Could you check a few things on this model? Use its own coordinates, in mm. Face numbers are marked on the shaded views. A direction names the side the tool comes from. Coordinates: 2 decimals unless noted, no trailing zeros. Write each loop counter-clockwise with the first axis right and the second up, starting at its lowest first coordinate (ties: lowest second). Pieces come first, ordered by that corner, then holes. Notation, with made-up numbers: (17.5, 78.5) - (43.5, 78.5) arc R15 cw to (43.5, 98.5) - close; hole circle Ø5 at (14, 56). An arc over 180 degrees is marked (long way). Write item = value, one per line. Start each with the question number.
```python
from build123d import *

# Parameters (mm, degrees)
BOX007_W          = 4.3
BOX007_H          = 5
BOX007_DEPTH      = 2
CHAMFER001_SIZE   = 1.5
BOX006_W          = 4.3
BOX006_H          = 5
BOX006_DEPTH      = 2
CHAMFER_SIZE      = 1.5
BOX003_W          = 10
BOX003_H          = 10
BOX003_DEPTH      = 40
BOX002_W          = 10
BOX002_H          = 10
BOX002_DEPTH      = 40
CYLINDER010_R     = 3.5
CYLINDER010_DEPTH = 35.7
CYLINDER008_R     = 4.6
CYLINDER008_DEPTH = 22
CYLINDER006_R     = 1.85
CYLINDER006_DEPTH = 10
CYLINDER003_R     = 1.7
CYLINDER003_DEPTH = 50
CYLINDER002_R     = 1.7
CYLINDER002_DEPTH = 50
CYLINDER_R        = 1.5
CYLINDER_DEPTH    = 10
BOX001_W          = 10
BOX001_H          = 6
BOX001_DEPTH      = 3
FILLET_R          = 2.5
FILLET001_R       = 2.5
BOX_W             = 65
BOX_H             = 22
BOX_DEPTH         = 18.5


with BuildPart() as chamfer001:
    # Box007 → Box007 (new body)
    with BuildSketch(Plane(origin=(41, -2.5, 17.53), x_dir=(1, 0, 0), z_dir=(0, 0, 1))):
        with Locations((2.15, 2.5)):
            Rectangle(BOX007_W, BOX007_H)
    extrude(amount=BOX007_DEPTH)

    # Chamfer001
    chamfer001_edges = [chamfer001.edges().sort_by_distance(p)[0] for p in [
        (45.3, 0, 19.53),
    ]]
    chamfer(chamfer001_edges, length=CHAMFER001_SIZE)


with BuildPart() as part_mirroring:
    # Part__Mirroring: instance of Chamfer001
    add(chamfer001.part.mirror(Plane(origin=(0, 0, 0), x_dir=(0, 1, 0), z_dir=(0, 0, 1))))


with BuildPart() as part_mirroring_1:
    # Part__Mirroring placement: moved
    add(part_mirroring.part.moved(Location((0, 0, 18.4))))


with BuildPart() as fusion004:
    # Box006 → Box006 (new body)
    with BuildSketch(Plane(origin=(41, -2.5, 17.53), x_dir=(1, 0, 0), z_dir=(0, 0, 1))):
        with Locations((2.15, 2.5)):
            Rectangle(BOX006_W, BOX006_H)
    extrude(amount=BOX006_DEPTH)

    # Chamfer
    chamfer_edges = [fusion004.edges().sort_by_distance(p)[0] for p in [
        (45.3, 0, 19.53),
    ]]
    chamfer(chamfer_edges, length=CHAMFER_SIZE)

    # Fusion004: union Part__Mirroring
    add(part_mirroring_1.part)


with BuildPart() as cube003:
    # Box003 → Box003 (new body)
    with BuildSketch(Plane(origin=(-0.55, -5, 5), x_dir=(1, 0, 0), z_dir=(0, 0, 1))):
        with Locations((5, 5)):
            Rectangle(BOX003_W, BOX003_H)
    extrude(amount=BOX003_DEPTH)


with BuildPart() as cube002:
    # Box002 → Box002 (new body)
    with BuildSketch(Plane(origin=(11.75, -5, -11), x_dir=(1, 0, 0), z_dir=(0, 0, 1))):
        with Locations((5, 5)):
            Rectangle(BOX002_W, BOX002_H)
    extrude(amount=BOX002_DEPTH)


with BuildPart() as cut004:
    # Cylinder010 → Cylinder010 (new body)
    with BuildSketch(Plane(origin=(10.6, 0, -9), x_dir=(1, 0, 0), z_dir=(0, 0, 1))):
        Circle(CYLINDER010_R)
    extrude(amount=CYLINDER010_DEPTH)

    # Cut003: cut Cube002
    add(cube002.part, mode=Mode.SUBTRACT)

    # Cut004: cut Cube003
    add(cube003.part, mode=Mode.SUBTRACT)


with BuildPart() as cylinder004:
    # Cylinder008 → Cylinder008 (new body)
    with BuildSketch(Plane(origin=(10.6, 0, -2.8), x_dir=(1, 0, 0), z_dir=(0, 0, 1))):
        Circle(CYLINDER008_R)
    extrude(amount=CYLINDER008_DEPTH)


with BuildPart() as cylinder003:
    # Cylinder006 → Cylinder006 (new body)
    with BuildSketch(Plane(origin=(22, 0, 10.2), x_dir=(1, 0, 0), z_dir=(0, 0, 1))):
        Circle(CYLINDER006_R)
    extrude(amount=CYLINDER006_DEPTH)


with BuildPart() as cylinder002:
    # Cylinder003 → Cylinder003 (new body)
    with BuildSketch(Plane(origin=(31, -8.8, -25), x_dir=(1, 0, 0), z_dir=(0, 0, 1))):
        Circle(CYLINDER003_R)
    extrude(amount=CYLINDER003_DEPTH)


with BuildPart() as cylinder001:
    # Cylinder002 → Cylinder002 (new body)
    with BuildSketch(Plane(origin=(31, 8.8, -25), x_dir=(1, 0, 0), z_dir=(0, 0, 1))):
        Circle(CYLINDER002_R)
    extrude(amount=CYLINDER002_DEPTH)


with BuildPart() as cylinder:
    # Cylinder → Cylinder (new body)
    with BuildSketch(Plane(origin=(-2.8, 0, 3), x_dir=(1, 0, 0), z_dir=(0, 0, 1))):
        Circle(CYLINDER_R)
    extrude(amount=CYLINDER_DEPTH)


with BuildPart() as fillet001:
    # Box001 → Box001 (new body)
    with BuildSketch(Plane(origin=(-5, -3, 7), x_dir=(1, 0, 0), z_dir=(0, 0, 1))):
        with Locations((5, 3)):
            Rectangle(BOX001_W, BOX001_H)
    extrude(amount=BOX001_DEPTH)

    # Cut: cut Cylinder
    add(cylinder.part, mode=Mode.SUBTRACT)

    # Fillet
    fillet_edges = [fillet001.edges().sort_by_distance(p)[0] for p in [
        (-5, -3, 8.5),
    ]]
    fillet(fillet_edges, radius=FILLET_R)

    # Fillet001
    fillet001_edges = [fillet001.edges().sort_by_distance(p)[0] for p in [
        (-5, 3, 8.5),
    ]]
    fillet(fillet001_edges, radius=FILLET001_R)


with BuildPart() as motor:
    # Box → Box (new body)
    with BuildSketch(Plane(origin=(0, -11, 0), x_dir=(1, 0, 0), z_dir=(0, 0, 1))):
        with Locations((32.5, 11)):
            Rectangle(BOX_W, BOX_H)
    extrude(amount=BOX_DEPTH)

    # Fusion: union Fillet001
    add(fillet001.part)

    # Cut001: cut Cylinder001
    add(cylinder001.part, mode=Mode.SUBTRACT)

    # Cut002: cut Cylinder002
    add(cylinder002.part, mode=Mode.SUBTRACT)

    # Fusion001: union Cylinder003
    add(cylinder003.part)

    # Fusion002: union Cylinder004
    add(cylinder004.part)

    # Fusion003: union Cut004
    add(cut004.part)

    # Fusion006: union Fusion004
    add(fusion004.part)


with BuildPart() as motor_1:
    # Fusion006 placement: moved
    add(motor.part.moved(Location((-10.6, 0, 3))))


solid = motor_1.part
```
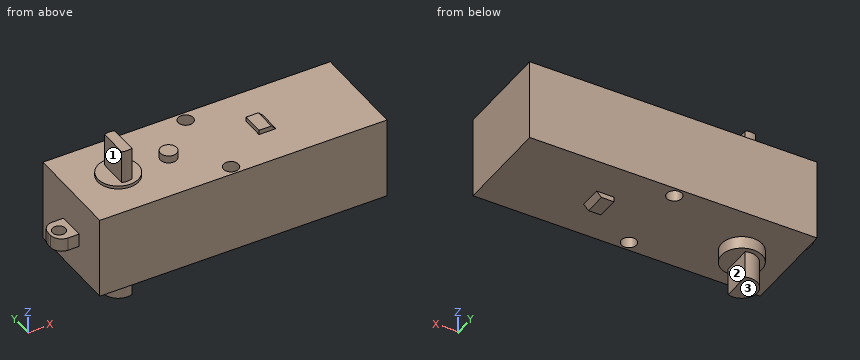
1) Suppose I cut it at A-A on y = -8.8. Please give me the cut outline in (x, z), plus the area to 3 significant figures.
2) If I drill on probe 1 along Y at (x, z) = (20.4, 10.5); probe 2 along X at (y, z) = (-8.8, 9); probe 3 along Z at (x, y) = (24, -8.5), over which ranges is the centre line in solid material (lowest first)? Write a range as [from, to].
3) Suppose I cut it at C-C on z = 7. Please give me the cut outline in (x, y), plus the area to 3 significant figures.
4) Which directions (+Z, -Z, +X, -X, +Y, -Y) give clear straight access to the entire face, cutting with the end or side of a thin tool? Please do the marked faces 1, 2 and 3.
5) For P1, Ø0.9, axis at x = 31.5, z = 2.5, coming from the -Y side; P2, Ø0.6, axis at x = 32.5, z = 2.5, coming from the +Y side; P3, Ø1.5, axis at x = 9, y = -1.5, coming from the +Z side, each with a flat end and sliding along its axis, tell me the tip position at first contact or that it passes through.
6) Suppose I cut it at D-D on x = 0. Please give me the cut outline in (y, z).
7) Suppose I cut it at B-B on x = 20.4. Please give me the cut outline in (y, z).
Reply:
q1.outline = (-10.6, 3) - (18.7, 3) - (18.7, 21.5) - (-10.6, 21.5) - close; (22.1, 3) - (54.4, 3) - (54.4, 21.5) - (22.1, 21.5) - close
q1.area = 1,140 mm^2
q2.probe_1 = [-11, -10.5], [-7.1, 7.1], [10.5, 11]
q2.probe_2 = [-10.6, 18.7], [22.1, 54.4]
q2.probe_3 = [3, 21.5]
q3.outline = (-10.6, -11) - (54.4, -11) - (54.4, 11) - (-10.6, 11) - close; hole circle Ø3.4 at (20.4, -8.8); hole circle Ø3.4 at (20.4, 8.8)
q3.area = 1,410 mm^2
q4.face_1 = +Z, -X, +Y, -Y
q4.face_2 = -Z, +X, +Y, -Y
q4.face_3 = -Z, +X, -X, +Y, -Y
q5.P1 = -2.5
q5.P2 = 2.5
q5.P3 = 21.5
q6.outline = (-11, 3) - (-4.6, 3) - (-4.6, 0.2) - (-3.5, 0.2) - (-3.5, -6) - (3.5, -6) - (3.5, 0.2) - (4.6, 0.2) - (4.6, 3) - (11, 3) - (11, 21.5) - (4.6, 21.5) - (4.6, 22.2) - (3.5, 22.2) - (3.5, 29.7) - (-3.5, 29.7) - (-3.5, 22.2) - (-4.6, 22.2) - (-4.6, 21.5) - (-11, 21.5) - close
q7.outline = (-11, 3) - (-10.5, 3) - (-10.5, 21.5) - (-11, 21.5) - close; (-7.1, 3) - (7.1, 3) - (7.1, 21.5) - (-7.1, 21.5) - close; (10.5, 3) - (11, 3) - (11, 21.5) - (10.5, 21.5) - close
